Can you work these out from the model? Positions are in its coordinate system, mm. Face numbers are marked on the shaded views. A direction names the side the tool comes from. Round coordinates to 2 decimals unless told otherwise and drop trailing zeros. Loops run counter-clockwise (first coordinate to the right, second up) from the corner with the lowest first, then second, coordinate; pieces in that order, holes last. Notation, with made-up numbers: M -38,-35 L 7,-35 A33 cw 7,1 Z; hole C -24,-3.75 d10. An arc over 180 degrees is marked long. Answer as CSV lines item,"result".
from build123d import *

# Parameters (mm, degrees)
SKETCH1_W           = 25.4
SKETCH1_H           = 50.8
SKETCH1_W_2         = 19.05
SKETCH1_H_2         = 44.45
BOSS_EXTRUDE1_DEPTH = 152.4
SKETCH2_R           = 2.5527
CUT_EXTRUDE1_DEPTH  = 50.8
SKETCH3_R           = 9.525
CUT_EXTRUDE2_DEPTH  = 25.4


with BuildPart() as part:
    # Sketch1 → Boss-Extrude1 (new body)
    with BuildSketch(Plane(origin=(0, 0, 0), x_dir=(1, 0, 0), z_dir=(0, 1, 0))):
        with Locations((12.7, 25.4)):
            Rectangle(SKETCH1_W, SKETCH1_H)
        with Locations((12.7, 25.4)):
            Rectangle(SKETCH1_W_2, SKETCH1_H_2, mode=Mode.SUBTRACT)
    extrude(amount=BOSS_EXTRUDE1_DEPTH)

    # Sketch2 → Cut-Extrude1 (cut)
    with BuildSketch(Plane(origin=(25.4, 0, 0), x_dir=(0, 0, -1), z_dir=(1, 0, 0))):
        with Locations((25.4, 139.7)):
            Circle(SKETCH2_R)
        with Locations((12.7, 114.3)):
            Circle(SKETCH2_R)
        with Locations((38.1, 114.3)):
            Circle(SKETCH2_R)
        with Locations((25.4, 41.275)):
            Circle(SKETCH2_R)
        with Locations((12.7, 15.875)):
            Circle(SKETCH2_R)
        with Locations((38.1, 15.875)):
            Circle(SKETCH2_R)
    extrude(amount=-CUT_EXTRUDE1_DEPTH, mode=Mode.SUBTRACT)

    # Sketch3 → Cut-Extrude2 (cut)
    with BuildSketch(Plane(origin=(25.4, 0, 0), x_dir=(0, 0, -1), z_dir=(1, 0, 0))):
        with Locations((25.4, 25.4)):
            Circle(SKETCH3_R)
    extrude(amount=-CUT_EXTRUDE2_DEPTH, mode=Mode.SUBTRACT)


solid = part.part
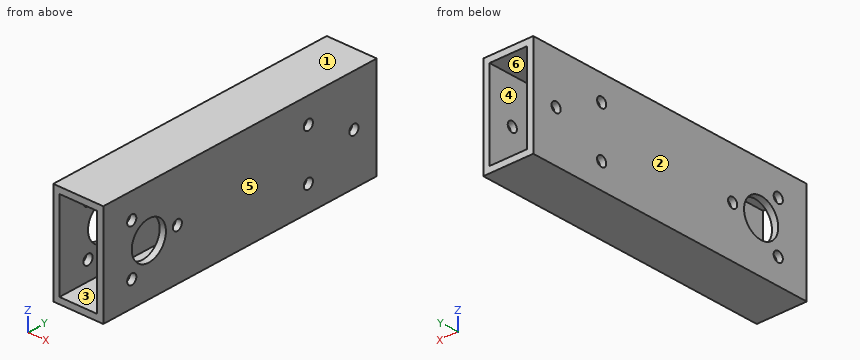
Item 1: We'd pull the mould along Z, two halves only. Please class the marked faces 1, 2, 3 and 4: released by +Z, released by -Z, zero draft, split by the parting line, or undercut.
Output:
face 1,"released by +Z"
face 2,"zero draft"
face 3,"undercut"
face 4,"undercut"
Item 2: If I drill on line 1 along Y through (x, z) = (1.2, -25.4) (3 decimals); line 2 along Y through (x, z) = (1.65, -12.7); line 3 along Z through (x, y) = (15.75, 116) (3 decimals), over which ranges is the centre line in solid material (lowest first)? Write a range as from..to.
Output:
line 1,"y = 0..15.875, 34.925..38.722, 43.828..137.147, 142.253..152.4"
line 2,"y = 0..13.32, 18.43..111.75, 116.85..152.4"
line 3,"z = -50.8..-47.625, -3.175..0"
Item 3: If we section it at D-D on y = 114.3: Write out the boundary of the cut face in (x, z) (3 decimals), then the cut area to 3 significant figures.
Output:
outline,"M 0,-50.8 L 25.4,-50.8 L 25.4,-40.653 L 22.225,-40.653 L 22.225,-47.625 L 3.175,-47.625 L 3.175,-40.653 L 0,-40.653 Z; M 0,-35.547 L 3.175,-35.547 L 3.175,-15.253 L 0,-15.253 Z; M 0,-10.147 L 3.175,-10.147 L 3.175,-3.175 L 22.225,-3.175 L 22.225,-10.147 L 25.4,-10.147 L 25.4,0 L 0,0 Z; M 22.225,-35.547 L 25.4,-35.547 L 25.4,-15.253 L 22.225,-15.253 Z"
area,"379 mm2"
Item 4: On a 3-axis mill with a long thin cutter (end or side, diameter ignored), from which of +Z, -Z, +X, -X, +Y, -Y can I reach the whole of each face in a straight line? I mean the marked faces 5 and 6. Say none if no direction works.
Output:
face 5,"+Z, -Z, +X, +Y, -Y"
face 6,"+Y, -Y"
Item 5: If we section it at C-C on z = -38.1: Write out the boundary of the cut face in (x, y) (3 decimals), then the cut area to 3 significant figures.
Output:
outline,"M 0,0 L 3.175,0 L 3.175,13.322 L 0,13.322 Z; M 0,18.428 L 3.175,18.428 L 3.175,111.747 L 0,111.747 Z; M 0,116.853 L 3.175,116.853 L 3.175,152.4 L 0,152.4 Z; M 22.225,0 L 25.4,0 L 25.4,13.322 L 22.225,13.322 Z; M 22.225,18.428 L 25.4,18.428 L 25.4,111.747 L 22.225,111.747 Z; M 22.225,116.853 L 25.4,116.853 L 25.4,152.4 L 22.225,152.4 Z"
area,"903 mm2"
Item 6: If we section it at B-B on y = 139.7: Write out the boundary of the cut face in (x, z) (3 decimals), then the cut area to 3 significant figures.
Output:
outline,"M 0,-50.8 L 25.4,-50.8 L 25.4,-27.953 L 22.225,-27.953 L 22.225,-47.625 L 3.175,-47.625 L 3.175,-27.953 L 0,-27.953 Z; M 0,-22.847 L 3.175,-22.847 L 3.175,-3.175 L 22.225,-3.175 L 22.225,-22.847 L 25.4,-22.847 L 25.4,0 L 0,0 Z"
area,"411 mm2"
Item 7: If we section it at A-A on x = 5.25: Write out the boundary of the cut face in (y, z) (3 decimals), then the cut area to 3 significant figures.
Output:
outline,"M 0,-50.8 L 152.4,-50.8 L 152.4,-47.625 L 0,-47.625 Z; M 0,-3.175 L 152.4,-3.175 L 152.4,0 L 0,0 Z"
area,"968 mm2"
